```python
from build123d import *

# Parameters (mm, degrees)
SKETCH1_W           = 100
SKETCH1_H           = 110
BOSS_EXTRUDE1_DEPTH = 130
SKETCH2_R           = 47.5
BOSS_EXTRUDE2_DEPTH = 50
SKETCH4_R           = 10
CUT_EXTRUDE3_DEPTH  = 20
SKETCH5_R           = 10
CUT_EXTRUDE4_DEPTH  = 20
FILLET1_R           = 5


with BuildPart() as part:
    # Sketch1 → Boss-Extrude1 (new body)
    with BuildSketch(Plane.XY):
        Rectangle(SKETCH1_W, SKETCH1_H)
    extrude(amount=BOSS_EXTRUDE1_DEPTH)

    # Sketch2 → Boss-Extrude2 (add)
    with BuildSketch(Plane(origin=(0, -55, 0), x_dir=(1, 0, 0), z_dir=(0, 1, 0))):
        with Locations(Location((0, -65, 0), (0, 0, 180))):
            Circle(SKETCH2_R)
    extrude(amount=-BOSS_EXTRUDE2_DEPTH)

    # Sketch4 → Cut-Extrude3 (cut)
    with BuildSketch(Plane.XZ.offset(105)):
        with Locations(Location((0, 65, 0), (0, 0, 270))):
            Circle(SKETCH4_R)
    extrude(amount=-CUT_EXTRUDE3_DEPTH, mode=Mode.SUBTRACT)

    # Sketch5 → Cut-Extrude4 (cut)
    with BuildSketch(Plane.XY.offset(130)):
        Circle(SKETCH5_R)
    extrude(amount=-CUT_EXTRUDE4_DEPTH, mode=Mode.SUBTRACT)

    # Fillet1
    fillet1_edges = [part.edges().sort_by_distance(p)[0] for p in [
        (50, 0, 130),
        (-50, 0, 130),
        (0, 55, 0),
        (50, 0, 0),
        (-50, 0, 0),
        (-50, 55, 65),
        (50, 55, 65),
    ]]
    fillet(fillet1_edges, radius=FILLET1_R)


solid = part.part
```
Part model, mm, in its own coordinate system. A direction names the side the tool comes from. Coordinates: 2 decimals unless noted, no trailing zeros. Write each loop counter-clockwise with the first axis right and the second up, starting at its lowest first coordinate (ties: lowest second). Pieces come first, ordered by that corner, then holes.
Item 1: Slice it at D-D (y = -90.5). Write the cut outline in (x, z), and give its area (3 significant figures).
Item 2: Pin check, flat tips, straight feed: pin 1 (4 mm diameter, centred on x = 7, y = -87.5, fed in from +Z); pin 2 (12 mm diameter, centred on x = 0, z = 65, fed in from -Y). Stop position of each tip, or through.
Item 3: Probe line 1 (Y direction, x = 0, z = 116.25); line 2 (Y direction, x = 3.5, z = 118); line 3 (Y direction, x = 36, z = 33). List the from-to ranges inside material, lowest first.
Item 4: Slice it at A-A (x = 0). Write the cut outline in (y, z).
Item 5: Mould opens along Y. For faces 1 (the face through (0, 0, 110)), 2 (the face through (-1, 55, 67)), 3 (the face through (0, -85, 65)), 4 (the face through (0, -95, 75)) say: released by +Y, released by -Y, zero draft, split by the parting line, or undercut.
Item 6: Which spindle directions (+Z, -Z, +X, -X, +Y, -Y) get a long thin tool onto all of the face, cutting with end or side? Do faces 5 (the face through (48, 54, 68)), 6 (the face through (-45.1, -55, 49.6)), 7 (the face through (-2.17, -9.76, 120.14)). Say none if no direction does.
Item 7: Slice it at B-B (y = 0). Write the cut outline in (x, z), and give its area (3 significant figures).
Item 8: Slice it at C-C (z = 65). Write the cut outline in (x, y), and give its area (3 significant figures).
Results found:
1. outline: circle Ø95 at (0, 65); hole circle Ø20 at (0, 65)
1. area: 6,770 mm2
2. pin 1: stops at z = 112.24
2. pin 2: stops at y = -85
3. line 1: y = -55 to -10, 10 to 55
3. line 2: y = -55 to -9.37, 9.37 to 55
3. line 3: y = -55 to 55
4. outline: (-105, 17.5) - (-55, 17.5) - (-55, 0) - (50, 0) arc R5 ccw to (55, 5) - (55, 130) - (10, 130) - (10, 110) - (-10, 110) - (-10, 130) - (-55, 130) - (-55, 112.5) - (-105, 112.5) - (-105, 75) - (-85, 75) - (-85, 55) - (-105, 55) - close
5. face 1: undercut
5. face 2: released by +Y
5. face 3: released by -Y
5. face 4: zero draft
6. face 5: +Z, -Z, +X, +Y
6. face 6: -Y
6. face 7: +Z
7. outline: (-50, 5) arc R5 ccw to (-45, 0) - (45, 0) arc R5 ccw to (50, 5) - (50, 125) arc R5 ccw to (45, 130) - (10, 130) - (10, 110) - (-10, 110) - (-10, 130) - (-45, 130) arc R5 ccw to (-50, 125) - close
7. area: 12,600 mm2
8. outline: (-50, -55) - (-47.5, -55) - (-47.5, -105) - (-10, -105) - (-10, -85) - (10, -85) - (10, -105) - (47.5, -105) - (47.5, -55) - (50, -55) - (50, 50) arc R5 ccw to (45, 55) - (-45, 55) arc R5 ccw to (-50, 50) - close
8. area: 15,300 mm2
